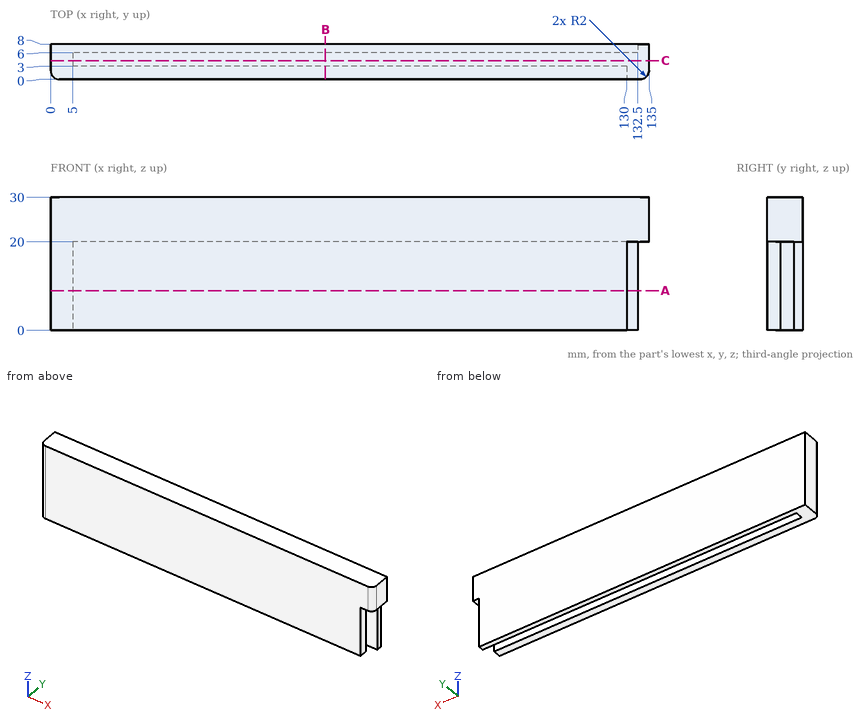
Job drawing, mm, ordinate dimensions from the low corner. One solid piece. Give positions to 0.01 mm unless a question says otherwise; leave off trailing zeros. Loops run counter-clockwise (first coordinate to the right, second up) from the corner with the lowest first, then second, coordinate; pieces in that order, holes last. Notation, with made-up numbers: M -14,13.5 L 18,13.5 A17 ccw 18,22.5 Z; hole C -37.5,-29.75 d6. An arc over 180 degrees is marked long. Answer in a Markdown table with one row per item. Add a question column.
Item 1: Drop flat-ended pins along their axis: P1, Ø3.5, axis at y = 1, z = 12.5, coming from the +X side; P2, Ø1, axis at y = 6.5, z = 11, coming from the +X side. Give the stop position or say it passes through.
Item 2: Band-saw the part on B-B on x = 62. Give the cut face in (y, z), then the cut area to 3 significant figures.
Item 3: Band-saw the part on C-C on y = 4.25. Give the cut face in (x, z).
Item 4: Probe probe 1 along Y at (x, z) = (68, 7.25); probe 2 along Z at (x, y) = (19, 5); probe 3 along X at (y, z) = (4.5, 2.5). List the from-to ranges inside material, lowest first.
Item 5: Band-saw the part on A-A on z = 9. Give the cut face in (x, y), then the cut area to 3 significant figures.
Reply:
| question | item | result |
|---|---|---|
| 1 | P1 | stops at x = 130 |
| 1 | P2 | stops at x = 132.5 |
| 2 | outline | M 0,0 L 3,0 L 3,20 L 6,20 L 6,0 L 8,0 L 8,30 L 0,30 Z |
| 2 | area | 180 mm^2 |
| 3 | outline | M 0,0 L 5,0 L 5,20 L 135,20 L 135,30 L 0,30 Z |
| 4 | probe 1 | y = 0 to 3, 6 to 8 |
| 4 | probe 2 | z = 20 to 30 |
| 4 | probe 3 | x = 0 to 5 |
| 5 | outline | M 0,2 A2 ccw 2,0 L 130,0 L 130,3 L 5,3 L 5,6 L 132.5,6 L 132.5,8 L 0,8 Z |
| 5 | area | 669 mm^2 |
